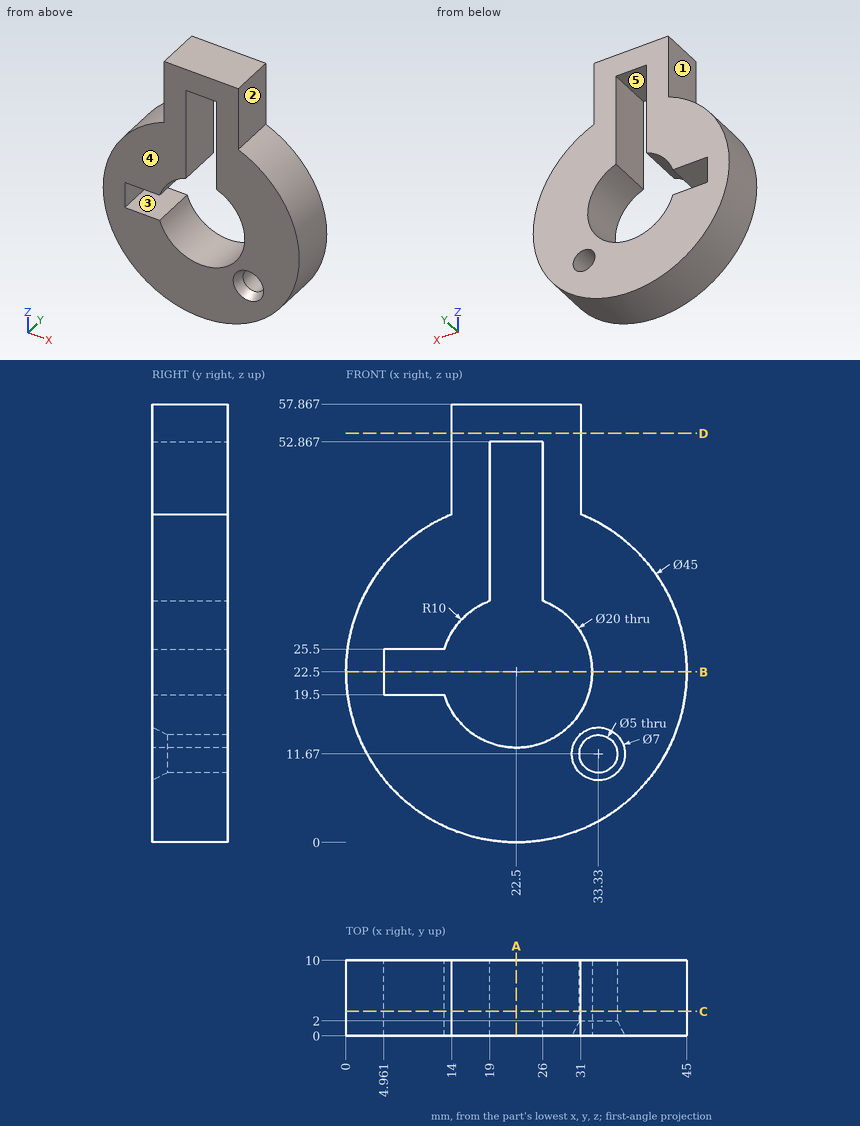
Print and shaded views of the part. All mm, measured from the part's lowest x, y and z. A direction names the side the tool comes from. Give positions to 0.01 mm unless a question says otherwise; leave off trailing zeros. Write each loop counter-clockwise with the first axis right and the second up, starting at its lowest first coordinate (ties: lowest second). Pieces come first, ordered by that corner, then holes. Notation, with made-up numbers: (15.25, 33.25) -> (46.25, 33.25) arc R26 ccw to (46.25, 66.25) -> close; hole circle Ø7 at (23.25, -26). An arc over 180 degrees is marked (long way). Use CSV: the item, a comma, the result in double quotes. Start each with the question number.
1) Tool access for the marked faces 4 and 5: list every direction of +Z, -Z, +X, -X, +Y, -Y with a clear straight run to the whole face (end or side of a thin tool).
2) Drill centre lines: L1, parallel to X at y = 4, z = 22.5; L2, parallel to X at y = 5, z = 52; L3, parallel to Z at x = 22, y = 1 (1 decimal). Where is each one in solid material? Low to high.
3) Pin check, flat tips, straight feed: P1, Ø5, axis at y = 6, z = 41.5, coming from the +X side (1 decimal); P2, Ø4, axis at x = 8, y = 6, coming from the +Z side; P3, Ø3, axis at y = 8, z = 46, coming from the +X side. Stop position of each tip, or through.
4) Cut at C-C on y = 3.25. List the corners of the cut face in (x, z).
5) Two-plate mould, pull along X, no slides. Class the marked faces 1, 2 and 3: released by +X, released by -X, zero draft, split by the parting line, or undercut.
6) Cut at D-D on z = 54. List the corners of the cut face in (x, y).
7) Cut at B-B on z = 22.5. List the corners of the cut face in (x, y), plus the area to 3 significant figures.
8) Cut at A-A on x = 22.5. List the corners of the cut face in (y, z).
Final values:
1,face 4,"+Z, -Z, +X, -X, -Y"
1,face 5,"+Y, -Y"
2,L1,"x = 0 to 4.96, 32.5 to 45"
2,L2,"x = 14 to 19, 26 to 31"
2,L3,"z = 0 to 12.5, 52.9 to 57.9"
3,P1,"stops at x = 37.8"
3,P2,"stops at z = 41.21"
3,P3,"stops at x = 31"
4,outline,"(14, 43.33) arc R22.5 ccw (long way) to (31, 43.33) -> (31, 57.87) -> (14, 57.87) -> close; hole (4.96, 19.5) -> (12.96, 19.5) arc R10 ccw (long way) to (26, 31.87) -> (26, 52.87) -> (19, 52.87) -> (19, 31.87) arc R10 ccw to (12.96, 25.5) -> (4.96, 25.5) -> close; hole circle Ø5 at (33.33, 11.67)"
5,face 1,"released by -X"
5,face 2,"released by +X"
5,face 3,"undercut"
6,outline,"(14, 0) -> (31, 0) -> (31, 10) -> (14, 10) -> close"
7,outline,"(0, 0) -> (4.96, 0) -> (4.96, 10) -> (0, 10) -> close; (32.5, 0) -> (45, 0) -> (45, 10) -> (32.5, 10) -> close"
7,area,"175 mm2"
8,outline,"(0, 0) -> (10, 0) -> (10, 12.5) -> (0, 12.5) -> close; (0, 52.87) -> (10, 52.87) -> (10, 57.87) -> (0, 57.87) -> close"
